```python
from build123d import *

# Parameters (mm, degrees)
FILLET1_R          = 1
SKETCH2_R          = 2.5
CUT_EXTRUDE1_DEPTH = 33.787192789


with BuildPart() as part:
    # Sketch1 → Revolve1 (revolve)
    with BuildSketch(Plane.XY, mode=Mode.PRIVATE) as revolve1_sk:
        with BuildLine():
            Line((-15, 19), (-15, -4))
            Line((-15, -4), (-12, -4))
            Line((-12, -4), (-12, 16))
            Line((-12, 16), (-5, 16))
            Line((-5, 16), (-5, 0))
            Line((-5, 0), (0, 0))
            Line((0, 0), (0, 21))
            ThreePointArc((0, 21), (-7.554204313, 20.406532346), (-15, 19))
        make_face()
    revolve(revolve1_sk.sketch.rotate(Axis((0, 0, 0), (0, 1, 0)), 270), axis=Axis((0, 0, 0), (0, 1, 0)))

    # Fillet1
    fillet1_edges = [part.edges().sort_by_distance(p)[0] for p in [
        (0, 19, 15),
    ]]
    fillet(fillet1_edges, radius=FILLET1_R)

    # Sketch2 → Cut-Extrude1 (cut, through all)
    with BuildSketch(Plane.XZ.offset(4)):
        with Locations((-17, 0)):
            Circle(SKETCH2_R)
        with Locations((-12.02081528, 12.02081528)):
            Circle(SKETCH2_R)
        with Locations((0, 17)):
            Circle(SKETCH2_R)
        with Locations((12.02081528, 12.02081528)):
            Circle(SKETCH2_R)
        with Locations((17, 0)):
            Circle(SKETCH2_R)
        with Locations((12.02081528, -12.02081528)):
            Circle(SKETCH2_R)
        with Locations((0, -17)):
            Circle(SKETCH2_R)
        with Locations((-12.02081528, -12.02081528)):
            Circle(SKETCH2_R)
    extrude(amount=-CUT_EXTRUDE1_DEPTH, mode=Mode.SUBTRACT)


solid = part.part
```
Geometry: final body of the model. Coordinates: model frame, mm. A direction names the side the tool comes from. Coordinates: 2 decimals unless noted, no trailing zeros. Loops run counter-clockwise (first coordinate to the right, second up) from the corner with the lowest first, then second, coordinate; pieces in that order, holes last. Notation, with made-up numbers: (8, 82.25) -> (66, 82.25) arc R29 ccw to (66, 106.25) -> close; hole circle Ø10 at (6.25, 33). An arc over 180 degrees is marked (long way). Use a Markdown table: item, result. Add a question column.
(1) Line query: line 1 along X through (y, z) = (4, 0); line 2 along Z through (x, y) = (2.25, 2); line 3 along Z through (x, y) = (3.5, 3). Output: solid intervals per line, ascending.
(2) Section query B-B, the plane y = -2. Return loops of the section in (x, z), plus the area to 3 significant figures.
(3) Access query for faces 1 (the cylindrical face through (14.5, 7.4, 0)), 2 (the flat face through (0, 0, 0)). Directions: +Z, -Z, +X, -X, +Y, -Y. A direction counts if a zero-diameter tool reaches every point of the face in a straight line with its end or side. Return the directions, or none.
(4) Section query A-A, the plane y = 1.5. Return loops of the section in (x, z), plus the area to 3 significant figures.
(5) Pin query (flat end, axial travel): pin 1 Ø5 at (y, z) = (17.5, 2.5) entering from -X; pin 2 Ø6 at (x, z) = (5.5, 7) entering from +Y; pin 3 Ø1.5 at (x, z) = (-10.5, 6.5) entering from +Y; pin 4 Ø1.5 at (y, z) = (7.5, 9.5) entering from +X. Return the tip coordinate at first contact, or that it passes through.
(6) Mould query, pull axis X, two halves, no side actions, for faces 3 (the cylindrical face through (13.882, 6.95, -5.682)), 4 (the flat face through (-0.2, 16, -5.2)), 5 (the cylindrical face through (-13.882, 6.95, 5.682)). Classes: pulls with the +X half, pulls with the -X half, needs draft (parallel to the pull), parting line crosses it, or undercut.
Answer:
| question | item | result |
|---|---|---|
| 1 | line 1 | x = -14.5 to -12, -5 to 5, 12 to 14.5 |
| 1 | line 2 | z = -14.83 to -11.79, -4.47 to 4.47, 11.79 to 14.83 |
| 1 | line 3 | z = -14.59 to -11.48, -3.57 to 3.57, 11.48 to 14.59 |
| 2 | outline | (-14.93, -1.41) arc R15 ccw to (-11.56, -9.56) arc R2.5 cw to (-9.56, -11.56) arc R15 ccw to (-1.41, -14.93) arc R2.5 cw to (1.41, -14.93) arc R15 ccw to (9.56, -11.56) arc R2.5 cw to (11.56, -9.56) arc R15 ccw to (14.93, -1.41) arc R2.5 cw to (14.93, 1.41) arc R15 ccw to (11.56, 9.56) arc R2.5 cw to (9.56, 11.56) arc R15 ccw to (1.41, 14.93) arc R2.5 cw to (-1.41, 14.93) arc R15 ccw to (-9.56, 11.56) arc R2.5 cw to (-11.56, 9.56) arc R15 ccw to (-14.93, 1.41) arc R2.5 cw to start; hole circle Ø24 at (0, 0) |
| 2 | area | 247 mm^2 |
| 3 | face 1 | +X, +Y, -Y |
| 3 | face 2 | -Y |
| 4 | outline | (-14.93, -1.41) arc R15 ccw to (-11.56, -9.56) arc R2.5 cw to (-9.56, -11.56) arc R15 ccw to (-1.41, -14.93) arc R2.5 cw to (1.41, -14.93) arc R15 ccw to (9.56, -11.56) arc R2.5 cw to (11.56, -9.56) arc R15 ccw to (14.93, -1.41) arc R2.5 cw to (14.93, 1.41) arc R15 ccw to (11.56, 9.56) arc R2.5 cw to (9.56, 11.56) arc R15 ccw to (1.41, 14.93) arc R2.5 cw to (-1.41, 14.93) arc R15 ccw to (-9.56, 11.56) arc R2.5 cw to (-11.56, 9.56) arc R15 ccw to (-14.93, 1.41) arc R2.5 cw to start; circle Ø10 at (0, 0); hole circle Ø24 at (0, 0) |
| 4 | area | 325 mm^2 |
| 5 | pin 1 | stops at x = -14.93 |
| 5 | pin 2 | stops at y = 20.61 |
| 5 | pin 3 | stops at y = 19.75 |
| 5 | pin 4 | stops at x = 12.18 |
| 6 | face 3 | pulls with the +X half |
| 6 | face 4 | undercut |
| 6 | face 5 | pulls with the -X half |
